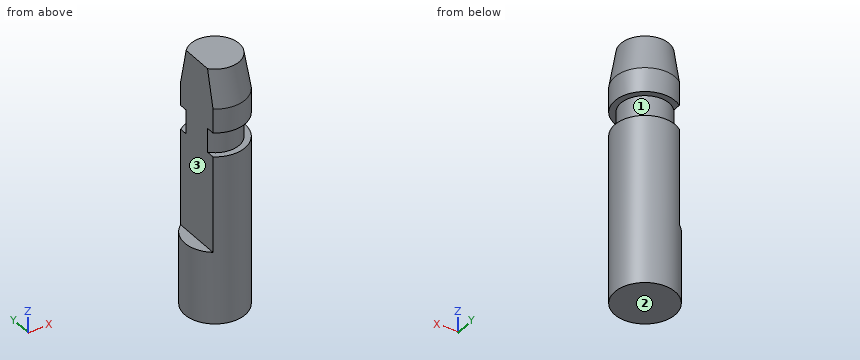
Autodesk Inventor part; units mm, degrees
ref_plane "Work Plane1" through (0, 0, 13.335) normal (0, 0, 1) x (1, 0, 0)
ref_plane "YZ Plane" through (0, 0, 0) normal (1, 0, 0) x (0, 1, 0)
ref_plane "XZ Plane" through (0, 0, 0) normal (0, 1, 0) x (-1, 0, 0)
sketch "Sketch1" plane through (0, 0, 0) normal (0, 0, 1) x (1, 0, 0)
  circle A0 centre (0, 0) radius 1.5875
  dimension "d0" = 3.175
extrude "Extrusion1" add sketch "Sketch1" along normal blind 3.81
sketch "Sketch2" plane through (0, 0, 3.81) normal (0, 0, 1) x (1, 0, 0)
  circle A0 centre (0, 0) radius 1.5875
  line L0 (-0.9525, 1.27) -> (-0.9525, -1.27)
  arc A1 (-0.9525, -1.27) -> (-0.9525, 1.27) centre (0, 0) ccw
  point P0 (1.5875, 0)
  point P1 (-0.9525, 0)
  dimension "d4" = 2.54
extrude "Extrusion2" add sketch "Sketch2" along normal blind 5.08 contours A0 L0 picked at (0.1068, 0.3913)
sketch "Sketch3" plane through (0, 0, 8.89) normal (0, 0, 1) x (1, 0, 0)
  arc A0 (-0.9525, -1.27) -> (-0.9525, 1.27) centre (0, 0) ccw
  line L0 (-0.9525, 1.27) -> (-0.9525, -1.27)
  arc A1 (-0.9525, -0.84) -> (-0.9525, 0.84) centre (0, 0) ccw
  line L1 (-0.9525, 0.84) -> (-0.9525, -0.84)
  dimension "d8" = 2.54
extrude "Extrusion3" add sketch "Sketch3" along normal blind 1.27 contours L0 A1
sketch "Sketch4" plane through (0, 0, 10.16) normal (0, 0, 1) x (1, 0, 0)
  line L0 (-0.9525, 0.84) -> (-0.9525, -0.84)
  arc A0 (-0.9525, -0.84) -> (-0.9525, 0.84) centre (0, 0) ccw
  arc A1 (-0.9525, -1.27) -> (-0.9525, 1.27) centre (0, 0) ccw
  line L1 (-0.9525, 1.27) -> (-0.9525, -1.27)
  dimension "d12" = 3.175
extrude "Extrusion4" add sketch "Sketch4" along normal blind 1.27
ref_plane "Work Plane1" through (0, 0, 13.335) normal (0, 0, 1) x (1, 0, 0)
sketch "Sketch5" plane through (0, 0, 13.335) normal (0, 0, 1) x (1, 0, 0)
  arc A0 (-0.9525, -0.84) -> (-0.9525, 0.84) centre (0, 0) ccw
  line L0 (-0.9525, 0.84) -> (-0.9525, -0.84)
  point P0 (1.5875, 0)
  point P1 (-0.9525, 0)
  dimension "d17" = 2.54
  dimension "d19" = 1.5875
  dimension "d20" = 2.54
sketch "Sketch6" plane through (0, 0, 11.43) normal (0, 0, 1) x (1, 0, 0)
  arc A0 (-0.9525, -1.27) -> (-0.9525, 1.27) centre (0, 0) ccw
  line L0 (-0.9525, 1.27) -> (-0.9525, -1.27)
loft "Loft1" add profiles "Sketch5" section 1 edges at (1.5875, 0, 11.43) (-0.9525, 0, 11.43)
properties part number "Lg Motor Shaft" material "Stainless Steel"
The listing builds one solid part. Answer for the finished solid, in the listing's coordinates (mm). Face numbers are marked on the shaded views. Round coordinates to 2 decimals unless told otherwise and drop trailing zeros. Write each loop counter-clockwise with the first axis right and the second up, starting at its lowest first coordinate (ties: lowest second). Pieces come first, ordered by that corner, then holes. Notation, with made-up numbers: (-33.75, 81) -> (23.25, 81) arc R4 cw to (23.25, 86) -> close; hole circle Ø9 at (-37, 43). An arc over 180 degrees is marked (long way). Answer as a JSON object with one key per item and string values. Group by question number.
Q1. Straight lines are drawn through the part: line 1 along Z through (x, y) = (-1, -0.35); line 2 along X through (y, z) = (0, 7.25); line 3 along Y through (x, z) = (0.95, 5). For each, find the intervals that lie inside material, in ascending order.
Q2. Determine the mould class of the marked faces 1, 2 and 3 for opening direction Z: pulls with the +Z half, pulls with the -Z half, needs draft (parallel to the pull), parting line crosses it, or undercut.
Q3. Section A-A (z = 4.5) is taken. Write down the section's boundary in (x, y) (1 decimal), plus the area to 3 significant figures.
Q4. Each of these flat-tipped pins is pushed along its axis until it touches: pin 1 Ø1.3 at (x, y) = (0, 0) entering from -Z; pin 2 Ø1.5 at (x, z) = (1, 3.5) entering from +Y; pin 3 Ø0.5 at (x, y) = (-1.5, -0.5) entering from +Z. Where does it stop, or does it pass through?
Check values:
{
 "1": {"line 1": "0 to 3.81", "line 2": "-0.95 to 1.59", "line 3": "-1.27 to 1.27"},
 "2": {"face 1": "undercut", "face 2": "pulls with the -Z half", "face 3": "needs draft"},
 "3": {"outline": "(-1, -1.3) arc R1.6 ccw (long way) to (-1, 1.3) -> close", "area": "6.79 mm^2"},
 "4": {"pin 1": "z = 0", "pin 2": "y = 1.57", "pin 3": "z = 3.81"}
}
